Work out the finished part from the listing and answer in its coordinate system (mm). A direction names the side the tool comes from. Give positions to 0.01 mm unless a question says otherwise; leave off trailing zeros. Loops run counter-clockwise (first coordinate to the right, second up) from the corner with the lowest first, then second, coordinate; pieces in that order, holes last. Notation, with made-up numbers: (69.5, 8.5) - (77.5, 8.5) arc R9 cw to (77.5, 16.5) - close; hole circle Ø6 at (-17.75, 39). An arc over 180 degrees is marked (long way). One line per item, written item: value.
from build123d import *

# Parameters (mm, degrees)
EXTRUDE_1_DEPTH             = 30
M3_TAPPED_HOLE1_D           = 2.5
M3_TAPPED_HOLE1_DEPTH       = 10
M3_TAPPED_HOLE1_CSINK_D     = 3.05
M3_TAPPED_HOLE1_CSINK_ANGLE = 90
M3_TAPPED_HOLE1_TIP         = 0.751075774
M3_TAPPED_HOLE2_D           = 2.5
M3_TAPPED_HOLE2_DEPTH       = 10
M3_TAPPED_HOLE2_CSINK_D     = 3.05
M3_TAPPED_HOLE2_CSINK_ANGLE = 90
M3_TAPPED_HOLE2_TIP         = 0.751075774


with BuildPart() as part:
    # 草图1 → 凸台-拉伸1 (new body)
    with BuildSketch(Plane(origin=(0, 0, 0), x_dir=(1, 0, 0), z_dir=(0, 1, 0))):
        Polygon((3.175426481, 0), (1.58771324, 2.75), (-1.58771324, 2.75), (-3.175426481, 0), (-1.58771324, -2.75), (1.58771324, -2.75), align=None)
    extrude(amount=EXTRUDE_1_DEPTH)

    # M3 Tapped Hole1
    with Locations(Plane(origin=(0, 30, 0), x_dir=(1, 0, 0), z_dir=(0, 1, 0))):
        with Locations((0, 0)):
            CounterSinkHole(M3_TAPPED_HOLE1_D / 2, M3_TAPPED_HOLE1_CSINK_D / 2, depth=M3_TAPPED_HOLE1_DEPTH, counter_sink_angle=M3_TAPPED_HOLE1_CSINK_ANGLE)
            with Locations((0, 0, -(M3_TAPPED_HOLE1_DEPTH + M3_TAPPED_HOLE1_TIP / 2))):  # 118° drill point
                Cone(0, M3_TAPPED_HOLE1_D / 2, M3_TAPPED_HOLE1_TIP, mode=Mode.SUBTRACT)

    # M3 Tapped Hole2
    with Locations(Plane(origin=(0, 0, 0), x_dir=(-1, 0, 0), z_dir=(0, -1, 0))):
        with Locations((0, 0)):
            CounterSinkHole(M3_TAPPED_HOLE2_D / 2, M3_TAPPED_HOLE2_CSINK_D / 2, depth=M3_TAPPED_HOLE2_DEPTH, counter_sink_angle=M3_TAPPED_HOLE2_CSINK_ANGLE)
            with Locations((0, 0, -(M3_TAPPED_HOLE2_DEPTH + M3_TAPPED_HOLE2_TIP / 2))):  # 118° drill point
                Cone(0, M3_TAPPED_HOLE2_D / 2, M3_TAPPED_HOLE2_TIP, mode=Mode.SUBTRACT)


solid = part.part
1. The mould has two halves that part along X. Classify faces 1 (the conical face through (-0.05, 19.38, 0.21)), 2 (the flat face through (2.37, 14.79, 1.394)), 3 (the flat face through (1.4, 0, 1.2)): released by +X, released by -X, zero draft, split by the parting line, or undercut.
Output:
face 1: undercut
face 2: released by +X
face 3: zero draft
2. Flat-ended cylindrical pins translate along their axes: pin 1 Ø3 at (x, z) = (0, 0) entering from -Y (3 decimals); pin 2 Ø2 at (x, z) = (0, 0) entering from +Y. Find the tip coordinate at first contact, or state that the pin passes through.
Output:
pin 1: stops at y = 0.025
pin 2: stops at y = 19.85
3. Section B-B (z = -1.8) is taken. Write down the section's boundary in (x, y).
Output:
outline: (-2.14, 0) - (2.14, 0) - (2.14, 30) - (-2.14, 30) - close
4. Find the intervals of material crossed by line 1 along Z through (x, y) = (0, 8.75); line 2 along X through (y, z) = (6.25, -0.5); line 3 along Z through (x, y) = (-1, 8.5), in increasing order.
Output:
line 1: z = -2.75 to -1.25, 1.25 to 2.75
line 2: x = -2.89 to -1.15, 1.15 to 2.89
line 3: z = -2.75 to -0.75, 0.75 to 2.75
5. Section C-C (x = -2) is taken. Write down the section's boundary in (y, z).
Output:
outline: (0, -2.04) - (30, -2.04) - (30, 2.04) - (0, 2.04) - close
6. Section A-A (y = 20.75) is taken. Write down the section's boundary in (x, z), and give its area (3 significant figures).
Output:
outline: (-3.18, 0) - (-1.59, -2.75) - (1.59, -2.75) - (3.18, 0) - (1.59, 2.75) - (-1.59, 2.75) - close; hole circle Ø2.5 at (0, 0)
area: 21.3 mm²
7. For faces 4 (the cylindrical face through (0.27, 24.79, 1.22)), 5 (the cylindrical face through (-0.27, 5.21, 1.22)), 6 (the flat face through (1.4, 30, 1.2)), determine the directions among +Z, -Z, +X, -X, +Y, -Y from which every point of the face is accessible in a straight line to the end or side of a thin tool.
Output:
face 4: +Y
face 5: -Y
face 6: +Z, -Z, +X, -X, +Y
